from build123d import *

# Parameters (mm, degrees)
BOX064_W          = 10
BOX064_H          = 10
BOX064_DEPTH      = 10
CYLINDER002_R     = 1
CYLINDER002_DEPTH = 9
CYLINDER001_R     = 1
CYLINDER001_DEPTH = 21
CYLINDER003_R     = 1
CYLINDER003_DEPTH = 10


with BuildPart() as box064:
    # Box064 → Box064 (new body)
    with BuildSketch(Plane(origin=(47, 14, 0), x_dir=(1, 0, 0), z_dir=(0, 0, 1))):
        with Locations((5, 5)):
            Rectangle(BOX064_W, BOX064_H)
    extrude(amount=BOX064_DEPTH)


with BuildPart() as cylinder002:
    # Cylinder002 → Cylinder002 (new body)
    with BuildSketch(Plane(origin=(47, 23, 7), x_dir=(1, 0, 0), z_dir=(0, 0, 1))):
        Circle(CYLINDER002_R)
    extrude(amount=CYLINDER002_DEPTH)


with BuildPart() as cut022:
    # Cylinder001 → Cylinder001 (new body)
    with BuildSketch(Plane(origin=(48, 23, 8), x_dir=(0, 0, 1), z_dir=(-1, 0, 0))):
        Circle(CYLINDER001_R)
    extrude(amount=CYLINDER001_DEPTH)

    # Cut021: cut Cylinder002
    add(cylinder002.part, mode=Mode.SUBTRACT)

    # Cut022: cut Box064
    add(box064.part, mode=Mode.SUBTRACT)


with BuildPart() as fusion025:
    # Cylinder003 → Cylinder003 (new body)
    with BuildSketch(Plane(origin=(47, 23, 7), x_dir=(1, 0, 0), z_dir=(0, 0, 1))):
        Circle(CYLINDER003_R)
    extrude(amount=CYLINDER003_DEPTH)

    # Fusion025: union Cut022
    add(cut022.part)


solid = fusion025.part
Check sheet for the modelled part. Datum: model origin and axes. Units: mm. A direction names the side the tool comes from. Give positions to 0.01 mm unless a question says otherwise; leave off trailing zeros. Write each loop counter-clockwise with the first axis right and the second up, starting at its lowest first coordinate (ties: lowest second). Pieces come first, ordered by that corner, then holes. Notation, with made-up numbers: (-20.75, 53.25) -> (2.25, 53.25) arc R20 cw to (2.25, 59.25) -> close; hole circle Ø6 at (-24, 31.5). An arc over 180 degrees is marked (long way). One line per item, written item: value. Start each with the question number.
Item 1: Section check A-A on y = 22.4. Record the cut outline in (x, z), then the cut area to 3 significant figures.
Item 2: Tool access check on faces 1 (the cylindrical face through (37, 23, 9)), 2 (the flat face through (47, 23, 7)). Record the directions out of +Z, -Z, +X, -X, +Y, -Y that give a thin tool (end or side, any length) a straight path to the whole face; none if there is none.
Item 3: Section check B-B on x = 34. Record the cut outline in (y, z).
Item 4: Section check C-C on z = 13.75. Record the cut outline in (x, y), then the cut area to 3 significant figures.
Item 5: Material ranges on probe 1 along X at (y, z) = (22.9, 16.5); probe 2 along Z at (x, y) = (39, 22.9); probe 3 along X at (y, z) = (22.4, 12.5), recorded low to high. Write a range as from..to.
Item 6: Section check D-D on y = 23.3. Record the cut outline in (x, z), then the cut area to 3 significant figures.
Item 7: Gauge pin test, flat ends, axial feed: pin 1 (3 mm diameter, centred on x = 30.5, z = 10, fed in from +Y); pin 2 (1 mm diameter, centred on y = 23.5, z = 12.5, fed in from +X). Record the tip position at first contact, or that the pin passes through.
Results list:
1. outline: (27, 7.2) -> (46.2, 7.2) -> (46.2, 7) -> (47.8, 7) -> (47.8, 17) -> (46.2, 17) -> (46.2, 8.8) -> (27, 8.8) -> close
1. area: 46.7 mm²
2. face 1: -X
2. face 2: -Z, +X, -X, +Y, -Y
3. outline: circle Ø2 at (23, 8)
4. outline: circle Ø2 at (47, 23)
4. area: 3.14 mm²
5. probe 1: 46.01..47.99
5. probe 2: 7.01..8.99
5. probe 3: 46.2..47.8
6. outline: (27, 7.05) -> (46.05, 7.05) -> (46.05, 7) -> (47.95, 7) -> (47.95, 17) -> (46.05, 17) -> (46.05, 8.95) -> (27, 8.95) -> close
6. area: 55.4 mm²
7. pin 1: y = 23.87
7. pin 2: x = 48
